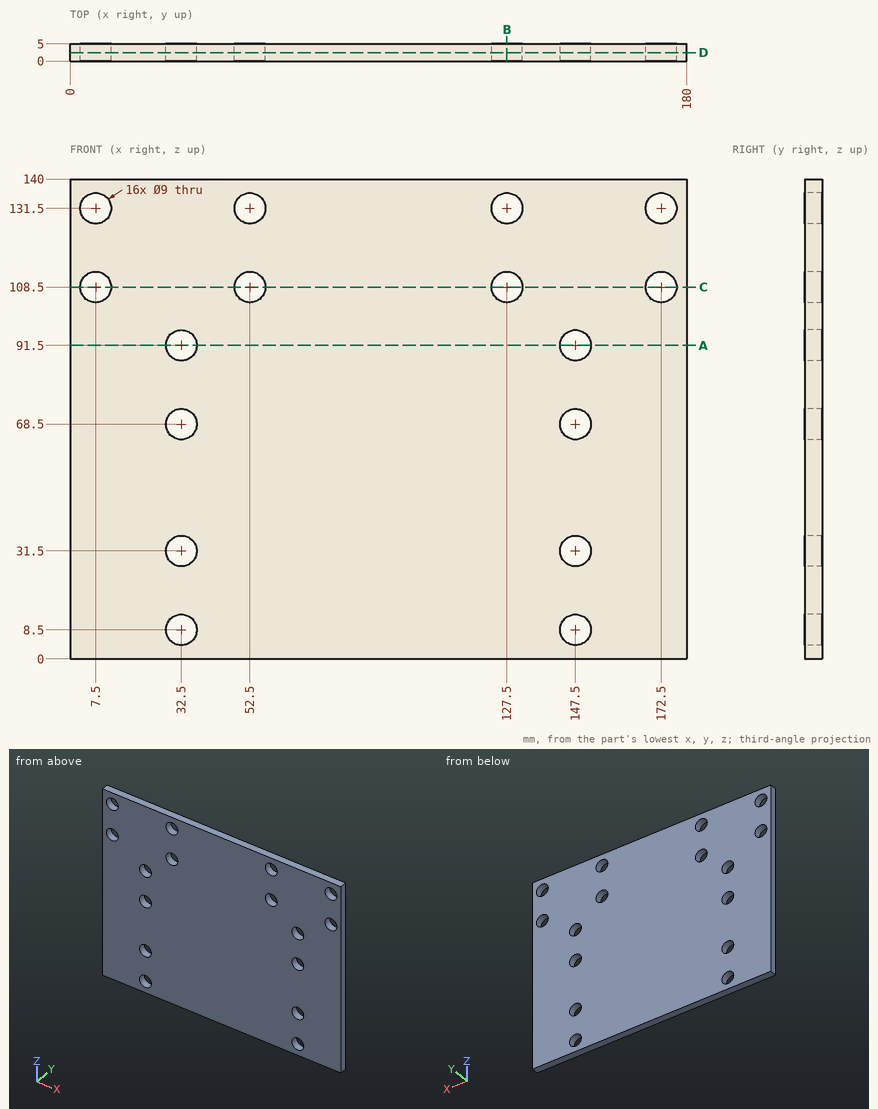
The drawing under review shows one solid part. Ordinate dimensions are in mm from its lowest x, y, z. Round coordinates to 2 decimals unless told otherwise and drop trailing zeros. Loops run counter-clockwise (first coordinate to the right, second up) from the corner with the lowest first, then second, coordinate; pieces in that order, holes last.
Item 1: Take a section at D-D (y = 2.5). Give the number of separate pieces and of enclosed holes in the cut face, then the cut area to 3 significant figures.
Determined:
separate pieces: 1
enclosed holes: 16
area: 24,200 mm2
Item 2: For line 1 (X direction, y = 1.85, z = 91.5); line 2 (Z direction, x = 147.5, y = 1.65); line 3 (X direction, y = 2.75, z = 131.5), list the stretches that pass through material, from the lowest coordinate up.
Determined:
line 1: x = 0 to 28, 37 to 143, 152 to 180
line 2: z = 0 to 4, 13 to 27, 36 to 64, 73 to 87, 96 to 140
line 3: x = 0 to 3, 12 to 48, 57 to 123, 132 to 168, 177 to 180
Item 3: Take a section at A-A (z = 91.5). Write out the cut boundary in (x, y), then the cut area to 3 significant figures.
Determined:
outline: (0, 0) - (28, 0) - (28, 5) - (0, 5) - close; (37, 0) - (143, 0) - (143, 5) - (37, 5) - close; (152, 0) - (180, 0) - (180, 5) - (152, 5) - close
area: 810 mm2
Item 4: Take a section at B-B (x = 127.5). Write out the cut boundary in (y, z), then the cut area to 3 significant figures.
Determined:
outline: (0, 0) - (5, 0) - (5, 104) - (0, 104) - close; (0, 113) - (5, 113) - (5, 127) - (0, 127) - close; (0, 136) - (5, 136) - (5, 140) - (0, 140) - close
area: 610 mm2
Item 5: Take a section at C-C (z = 108.5). Write out the cut boundary in (x, y), then the cut area to 3 significant figures.
Determined:
outline: (0, 0) - (3, 0) - (3, 5) - (0, 5) - close; (12, 0) - (48, 0) - (48, 5) - (12, 5) - close; (57, 0) - (123, 0) - (123, 5) - (57, 5) - close; (132, 0) - (168, 0) - (168, 5) - (132, 5) - close; (177, 0) - (180, 0) - (180, 5) - (177, 5) - close
area: 720 mm2
